Geometry: final body of the model. Coordinates: model frame, mm. Face numbers are marked on the shaded views. A direction names the side the tool comes from. Round coordinates to 2 decimals unless told otherwise and drop trailing zeros. Write each loop counter-clockwise with the first axis right and the second up, starting at its lowest first coordinate (ties: lowest second). Pieces come first, ordered by that corner, then holes. Notation, with made-up numbers: M -36,31.25 L -27,31.25 A21 cw -27,54.25 Z; hole C 21,27.25 d11. An arc over 180 degrees is marked long. Use one line per item in the form item = value. Start each with the question number.
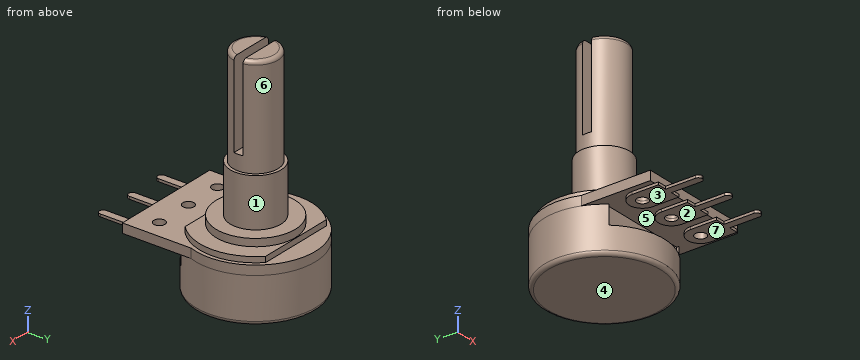
from build123d import *

# Parameters (mm, degrees)
F0_R      = 8
F1_DEPTH  = 6
F3_DEPTH  = 1.25
F5_DEPTH  = 0.75
F6_R      = 5.3
F7_DEPTH  = 1
F8_R      = 3.4
F9_DEPTH  = 6.5
F10_R     = 3
F11_DEPTH = 13.5
F12_W     = 12
F12_H     = 6
F13_DEPTH = 2.5
F14_R     = 0.75
F15_DEPTH = 25
F16_R     = 0.75
F17_DEPTH = 0.35
F18_R     = 0.5
F19_W     = 11.885716
F19_H     = 1.2
F20_DEPTH = 11.5


with BuildPart() as f1:
    # F0 (on Top) → F1 (new body)
    with BuildSketch(Plane.XY):
        Circle(F0_R)
    extrude(amount=F1_DEPTH)

    # F2 (on face) → F3 (join)
    with BuildSketch(Plane.XY.offset(6)):
        with BuildLine():
            Line((-7.5, -12), (7.5, -12))
            Line((7.5, -12), (7.5, -2.783882))
            ThreePointArc((7.5, -2.783882), (0, 8), (-7.5, -2.783882))
            Line((-7.5, -2.783882), (-7.5, -12))
        make_face()
    extrude(amount=F3_DEPTH)

    # F4 (on face) → F5 (join)
    with BuildSketch(Plane.XY.offset(7.25)):
        with BuildLine():
            Line((5.204805, 5.4), (-5.204805, 5.4))
            ThreePointArc((-5.204805, 5.4), (-7.5, 0), (-5.204805, -5.4))
            Line((-5.204805, -5.4), (5.204805, -5.4))
            ThreePointArc((5.204805, -5.4), (7.5, 0), (5.204805, 5.4))
        make_face()
    extrude(amount=F5_DEPTH)

    # F6 (on face) → F7 (join)
    with BuildSketch(Plane.XY.offset(8)):
        Circle(F6_R)
    extrude(amount=F7_DEPTH)

    # F8 (on face) → F9 (join)
    with BuildSketch(Plane.XY.offset(9)):
        Circle(F8_R)
    extrude(amount=F9_DEPTH)

    # F10 (on face) → F11 (join)
    with BuildSketch(Plane.XY.offset(15.5)):
        Circle(F10_R)
    extrude(amount=F11_DEPTH)

    # F12 (on face) → F13 (cut)
    with BuildSketch(Plane(origin=(0, 0, 6), x_dir=(1, 0, 0), z_dir=(0, 0, -1))):
        with Locations((0, 8)):
            Rectangle(F12_W, F12_H)
    extrude(amount=F13_DEPTH, mode=Mode.SUBTRACT)

    # F14 (on face) → F15 (cut)
    with BuildSketch(Plane.XY.offset(7.25)):
        with Locations((-5, -9)):
            Circle(F14_R)
        with Locations((0, -9)):
            Circle(F14_R)
        with Locations((5, -9)):
            Circle(F14_R)
    extrude(amount=-F15_DEPTH, mode=Mode.SUBTRACT)

    # F16 (on face) → F17 (join)
    with BuildSketch(Plane(origin=(0, 0, 6), x_dir=(1, 0, 0), z_dir=(0, 0, -1))):
        with BuildLine():
            Line((4.5, 12.5), (3.25, 12.5))
            Line((3.25, 12.5), (3.25, 9))
            ThreePointArc((3.25, 9), (5, 7.25), (6.75, 9))
            Line((6.75, 9), (6.75, 12.5))
            Line((6.75, 12.5), (5.5, 12.5))
            Line((5.5, 12.5), (5.5, 16.5))
            ThreePointArc((5.5, 16.5), (5.353553, 16.853553), (5, 17))
            ThreePointArc((5, 17), (4.646447, 16.853553), (4.5, 16.5))
            Line((4.5, 16.5), (4.5, 12.5))
        make_face()
        with Locations((5, 9)):
            Circle(F16_R, mode=Mode.SUBTRACT)
        with BuildLine():
            Line((-0.5, 16.5), (-0.5, 12.5))
            Line((-0.5, 12.5), (-1.75, 12.5))
            Line((-1.75, 12.5), (-1.75, 9))
            ThreePointArc((-1.75, 9), (0, 7.25), (1.75, 9))
            Line((1.75, 9), (1.75, 12.5))
            Line((1.75, 12.5), (0.5, 12.5))
            Line((0.5, 12.5), (0.5, 16.5))
            ThreePointArc((0.5, 16.5), (0.353553, 16.853553), (0, 17))
            ThreePointArc((0, 17), (-0.353553, 16.853553), (-0.5, 16.5))
        make_face()
        with Locations((0, 9)):
            Circle(F16_R, mode=Mode.SUBTRACT)
        with BuildLine():
            Line((-5.5, 16.5), (-5.5, 12.5))
            Line((-5.5, 12.5), (-6.75, 12.5))
            Line((-6.75, 12.5), (-6.75, 9))
            ThreePointArc((-6.75, 9), (-5, 7.25), (-3.25, 9))
            Line((-3.25, 9), (-3.25, 12.5))
            Line((-3.25, 12.5), (-4.5, 12.5))
            Line((-4.5, 12.5), (-4.5, 16.5))
            ThreePointArc((-4.5, 16.5), (-4.646447, 16.853553), (-5, 17))
            ThreePointArc((-5, 17), (-5.353553, 16.853553), (-5.5, 16.5))
        make_face()
        with Locations((-5, 9)):
            Circle(F16_R, mode=Mode.SUBTRACT)
    extrude(amount=F17_DEPTH)

    # F18
    f18_edges = [f1.edges().sort_by_distance(p)[0] for p in [
        (-3, 0, 29),
        (-8, 0, 0),
    ]]
    fillet(f18_edges, radius=F18_R)

    # F19 (on face) → F20 (cut)
    with BuildSketch(Plane.XY.offset(29)):
        Rectangle(F19_W, F19_H)
    extrude(amount=-F20_DEPTH, mode=Mode.SUBTRACT)


solid = f1.part
1. Section query B-B (y = 0). Return loops of the section in (x, z).
2. Ray query, probe 1 along X at (y, z) = (-9, 5.85); probe 2 along Z at (x, y) = (-3.25, -1.25); probe 3 along Y at (x, z) = (0, 6.4). Return the intervals inside material, ascending.
3. Contact query for flat-ended pins moving along their axis: pin 1 (1.5 mm diameter, centred on x = -3.5, z = 12.5, fed in from +Y); pin 2 (5 mm diameter, centred on y = 4.5, z = 8.5, fed in from +X); pin 3 (1 mm diameter, centred on x = 5.5, y = -7, fed in from +Z). Output: stop coordinate, or through.
4. Set-up query: the marked faces 1, 2, 3 and 4. Return all of +Z, -Z, +X, -X, +Y, -Y with unobstructed straight access to the full face (end or side cutting, diameter ignored); none if empty.
5. Section query A-A (y = -14.5). Return loops of the section in (x, z), then the cut area to 3 significant figures.
6. Section query C-C (z = 20). Return loops of the section in (x, y).
7. Pull-direction query (X, two-part tool) for the marked faces 5, 6 and 7; classes: released by +X, released by -X, zero draft, split by the parting line, or undercut.
8. Section query D-D (z = 8.5). Return loops of the section in (x, y).
Checks:
q1.outline = M -8,0.5 A0.5 ccw -7.5,0 L 7.5,0 A0.5 ccw 8,0.5 L 8,7.25 L 7.5,7.25 L 7.5,8 L 5.3,8 L 5.3,9 L 3.4,9 L 3.4,15.5 L 3,15.5 L 3,17.5 L -3,17.5 L -3,15.5 L -3.4,15.5 L -3.4,9 L -5.3,9 L -5.3,8 L -7.5,8 L -7.5,7.25 L -8,7.25 Z
q2.probe_1 = -6.75 to -5.75, -4.25 to -3.25, -1.75 to -0.75, 0.75 to 1.75, 3.25 to 4.25, 5.75 to 6.75
q2.probe_2 = 0 to 9
q2.probe_3 = -12 to -9.75, -8.25 to 8
q3.pin_1 = 2
q3.pin_2 = 7.65
q3.pin_3 = 7.25
q4.face_1 = +Z
q4.face_2 = +X, -X, -Y
q4.face_3 = -Z, +X, -X, -Y
q4.face_4 = -Z, +X, -X, +Y, -Y
q5.outline = M -5.5,5.65 L -4.5,5.65 L -4.5,6 L -5.5,6 Z; M -0.5,5.65 L 0.5,5.65 L 0.5,6 L -0.5,6 Z; M 4.5,5.65 L 5.5,5.65 L 5.5,6 L 4.5,6 Z
q5.area = 1.05 mm^2
q6.outline = M -2.94,-0.6 A3 ccw 2.94,-0.6 Z; M -2.94,0.6 L 2.94,0.6 A3 ccw Z
q7.face_5 = undercut
q7.face_6 = split by the parting line
q7.face_7 = zero draft
q8.outline = C 0,0 d10.6
